Work out the finished part from the listing and answer in its coordinate system (mm). A direction names the side the tool comes from. Coordinates: 2 decimals unless noted, no trailing zeros. Write each loop counter-clockwise with the first axis right and the second up, starting at its lowest first coordinate (ties: lowest second). Pieces come first, ordered by that corner, then holes. Notation, with made-up numbers: (56.5, -18) - (64.5, -18) arc R22 ccw to (64.5, -10) - close; hole circle Ø8 at (61, 60.25). An arc over 180 degrees is marked (long way). Use a Markdown table: item, result. Add a question column.
(1) For a pull along Z with two mould halves and no side action, classify faces 1 (the face through (-6, 43, 0)), 2 (the face through (-1.426, 43.009, 11.16)), 3 (the face through (-32, 31, 25)), 4 (the face through (-12.572, 32.377, 11.154)) as released by +Z, released by -Z, zero draft, split by the parting line, or undercut.
(2) The part is cut by section A-A, the plane x = -24. State how many separate pieces and enclosed holes the cut face has, then the cut area to 3 significant figures.
(3) The part is cut by section D-D, the plane y = 18. Give the vertices of the cut face in (x, z), then the cut area to 3 significant figures.
(4) The part is cut by section B-B, the plane y = 26. Give the vertices of the cut face in (x, z), then the cut area to 3 significant figures.
(5) Find the intervals of material crossed by line 1 (X direction, y = 20, z = 3.75); line 2 (X direction, y = 35, z = 10.5); line 3 (Z direction, x = -3, y = 7), in increasing order. Write a range as from..to.
(6) Given pin 1 Ø4 at (x, z) = (-37, 8.5) entering from +Y; pin 2 Ø10.5 at (x, y) = (-27.5, 13.5) entering from -Z; pin 3 Ø12 at (x, y) = (-8, 8) entering from +Z, each flat-ended and moving along its own axis, determine where each tip first touches the part or whether it passes through.
(7) A tool of negligible diameter and unlimited length cuts with its end or side. For faces 5 (the face through (-31.24, 38.67, 22.45)), 6 (the face through (-57, 42, 22)), 7 (the face through (-9.8, 44.11, 11.15)), 8 (the face through (-11, 12, 11)), 9 (the face through (-32, 31, 0)), from which of +Z, -Z, +X, -X, +Y, -Y can it reach the whole face along a straight path? Write none if from no direction.
from build123d import *

# Parameters (mm, degrees)
BOSS_EXTRUDE1_DEPTH = 22
FILLET2_R           = 5
FILLET4_R           = 5
FILLET5_R           = 1.5
FILLET6_R           = 3
FILLET7_R           = 1.5
SKETCH5_W           = 63
SKETCH5_H           = 16.840827273
BOSS_EXTRUDE2_DEPTH = 3
SKETCH6_W           = 63
SKETCH6_H           = 16.840827273
BOSS_EXTRUDE3_DEPTH = 3
FILLET8_R           = 1.5
FILLET9_R           = 1.5


with BuildPart() as part:
    # Sketch1 → Boss-Extrude1 (new body)
    with BuildSketch(Plane(origin=(0, 0, 0), x_dir=(0, 1, 0), z_dir=(0, 0, 1))):
        Polygon((0, 0), (44.512606441, 0), (44.512606441, 10), (39.512606441, 13), (31.925649919, 13), (31.925649919, 10), (10, 10), (10, 53), (31.925649919, 53), (31.925649919, 50), (39.512606441, 50), (44.512606441, 53), (44.512606441, 63), (0, 63), align=None)
    extrude(amount=BOSS_EXTRUDE1_DEPTH)

    # Fillet2
    fillet2_edges = [part.edges().sort_by_distance(p)[0] for p in [
        (-63, 0, 11),
        (-63, 44.512606441, 11),
        (0, 44.512606441, 11),
        (0, 0, 11),
    ]]
    fillet(fillet2_edges, radius=FILLET2_R)

    # Fillet4
    fillet4_edges = [part.edges().sort_by_distance(p)[0] for p in [
        (-53, 10, 11),
        (-10, 10, 11),
    ]]
    fillet(fillet4_edges, radius=FILLET4_R)

    # Fillet5
    fillet5_edges = [part.edges().sort_by_distance(p)[0] for p in [
        (-53, 31.925649919, 11),
        (-10, 31.925649919, 11),
    ]]
    fillet(fillet5_edges, radius=FILLET5_R)

    # Fillet6
    fillet6_edges = [part.edges().sort_by_distance(p)[0] for p in [
        (-53, 44.512606441, 11),
        (-10, 44.512606441, 11),
    ]]
    fillet(fillet6_edges, radius=FILLET6_R)

    # Fillet7
    fillet7_edges = [part.edges().sort_by_distance(p)[0] for p in [
        (-13, 39.512606441, 11),
        (-50, 39.512606441, 11),
        (-50, 31.925649919, 11),
        (-13, 31.925649919, 11),
    ]]
    fillet(fillet7_edges, radius=FILLET7_R - 0.0001)  # a hair under: the kernel refuses the full size

    # Sketch5 → Boss-Extrude2 (add)
    with BuildSketch(Plane.XY.offset(22)):
        with Locations((-31.5, 30.676716857)):
            Rectangle(SKETCH5_W, SKETCH5_H)
    extrude(amount=BOSS_EXTRUDE2_DEPTH)

    # Sketch6 → Boss-Extrude3 (add)
    with BuildSketch(Plane(origin=(0, 0, 0), x_dir=(1, 0, 0), z_dir=(0, 0, -1))):
        with Locations((-31.5, -30.676716857)):
            Rectangle(SKETCH6_W, SKETCH6_H)
    extrude(amount=BOSS_EXTRUDE3_DEPTH)

    # Fillet8
    fillet8_edges = [part.edges().sort_by_distance(p)[0] for p in [
        (-31.5, 22.25630322, 22),
        (-31.5, 39.097130493, 25),
        (-31.5, 22.25630322, 25),
        (-31.5, 39.097130493, 22),
        (-31.5, 39.097130493, 0),
        (-31.5, 22.25630322, 0),
        (-31.5, 39.097130493, -3),
        (-31.5, 22.25630322, -3),
    ]]
    fillet(fillet8_edges, radius=FILLET8_R - 0.0001)  # a hair under: the kernel refuses the full size

    # Fillet9
    fillet9_edges = [part.edges().sort_by_distance(p)[0] for p in [
        (-5, 22.25630322, 22),
    ]]
    fillet(fillet9_edges, radius=FILLET9_R - 0.0001)  # a hair under: the kernel refuses the full size
    fillet9_2_edges = [part.edges().sort_by_distance(p)[0] for p in [
        (-58, 22.25630322, 22),
    ]]
    fillet(fillet9_2_edges, radius=FILLET9_R - 0.0001)  # a hair under: the kernel refuses the full size
    fillet9_3_edges = [part.edges().sort_by_distance(p)[0] for p in [
        (-58, 22.25630322, 0),
    ]]
    fillet(fillet9_3_edges, radius=FILLET9_R - 0.0001)  # a hair under: the kernel refuses the full size
    fillet9_4_edges = [part.edges().sort_by_distance(p)[0] for p in [
        (-5, 22.25630322, 0),
    ]]
    fillet(fillet9_4_edges, radius=FILLET9_R - 0.0001)  # a hair under: the kernel refuses the full size
    fillet9_5_edges = [part.edges().sort_by_distance(p)[0] for p in [
        (-56.5, 39.097130493, 22),
    ]]
    fillet(fillet9_5_edges, radius=FILLET9_R - 0.0001)  # a hair under: the kernel refuses the full size
    fillet9_6_edges = [part.edges().sort_by_distance(p)[0] for p in [
        (-6.5, 39.097130493, 22),
    ]]
    fillet(fillet9_6_edges, radius=FILLET9_R - 0.0001)  # a hair under: the kernel refuses the full size
    fillet9_7_edges = [part.edges().sort_by_distance(p)[0] for p in [
        (-6.5, 39.097130493, 0),
    ]]
    fillet(fillet9_7_edges, radius=FILLET9_R - 0.0001)  # a hair under: the kernel refuses the full size
    fillet9_8_edges = [part.edges().sort_by_distance(p)[0] for p in [
        (-56.5, 39.097130493, 0),
    ]]
    fillet(fillet9_8_edges, radius=FILLET9_R - 0.0001)  # a hair under: the kernel refuses the full size


solid = part.part
Model answer:
| question | item | result |
|---|---|---|
| 1 | face 1 | released by -Z |
| 1 | face 2 | zero draft |
| 1 | face 3 | released by +Z |
| 1 | face 4 | undercut |
| 2 | separate pieces | 3 |
| 2 | enclosed holes | 0 |
| 2 | area | 317 mm^2 |
| 3 | outline | (-63, 0) - (-53, 0) - (-53, 22) - (-63, 22) - close; (-10, 0) - (0, 0) - (0, 22) - (-10, 22) - close |
| 3 | area | 440 mm^2 |
| 4 | outline | (-63, -3) - (0, -3) - (0, 25) - (-63, 25) - close; hole (-53, 0) - (-10, 0) - (-10, 22) - (-53, 22) - close |
| 4 | area | 818 mm^2 |
| 5 | line 1 | -63..-53, -10..0 |
| 5 | line 2 | -63..-50, -13..0 |
| 5 | line 3 | 0..22 |
| 6 | pin 1 | y = 10 |
| 6 | pin 2 | z = 0 |
| 6 | pin 3 | z = 22 |
| 7 | face 5 | +Y |
| 7 | face 6 | +Z, +X, -X, +Y |
| 7 | face 7 | +Z, -Z, +Y |
| 7 | face 8 | +Z, -Z |
| 7 | face 9 | none |
